Verification items for the finished model (mm, model axes). A direction names the side the tool comes from. Give positions to 0.01 mm unless a question says otherwise; leave off trailing zeros. Order: outer loops, then holes, each group sorted by start corner. A loop starts at its lowest first (then second) coordinate and runs counter-clockwise, first axis right, second up. Notation, with made-up numbers: (-6.5, 83.25) -> (-2.5, 83.25) arc R24 cw to (-2.5, 109.25) -> close; hole circle Ø9 at (-0.5, 12.5). An arc over 180 degrees is marked (long way). Write each question's results on one line, items separated by ' | '. Start each with the question number.
1. Cross-section at A-A, the plane y = 0. Enter the section's corners in (x, z) (3 decimals), then the cut area to 3 significant figures.
2. Material ranges on L1, parallel to Z at x = -12.5, y = -21.5; L2, parallel to X at y = -24.5, z = 62.5; L3, parallel to X at y = 35.5, z = 1, recorded low to high. Write a range as from..to.
3. Cross-section at B-B, the plane x = 30. Enter the section's corners in (y, z).
4. Depth check by flat-ended pin: pin 1 Ø16 at (y, z) = (0, 50.07) entering from +X; pin 2 Ø8 at (x, y) = (32, -9.5) entering from +Z; pin 3 Ø5 at (y, z) = (30, 75.07) entering from +X. Enter the tip coordinate at first touch or a pass-through.
5. Cross-section at C-C, the plane y = 30. Enter the section's corners in (x, z) (3 decimals), then the cut area to 3 significant figures.
6. Set-up check for faces 5 (the face through (-46.962, 9, 51)), 6 (the face through (2, 1, -3.038)): record each of +Z, -Z, +X, -X, +Y, -Y from which the full face is reachable in a straight line by a thin tool's end or side.
7. Mould release check, pull along X, two halves, no side actions. Record for faces 1 (the face through (-48.502, 22.968, 55.934)), 2 (the face through (-50, 9, 49)), 3 (the face through (26.746, -32.495, -1.498)), 4 (the face through (50, -1, -1)): +X half, -X half, draft (parallel to the pull), parting line (faces both ways), or undercut.
8. Cross-section at D-D, the plane y = 11.5. Enter the section's corners in (x, z) (3 decimals), then the cut area to 3 significant figures.
from build123d import *

# Parameters (mm, degrees)
CROQUIS1_W                       = 100
CROQUIS1_H                       = 80
CROQUIS1_R                       = 4.1
BRIDA_BASE1_DEPTH                = 3.03784
BRIDA_DE_ARISTA1_STRIP_W         = 18.50136
BRIDA_DE_ARISTA1_STRIP_H         = 3.03784
BRIDA_DE_ARISTA1_STRIP_CUT_DEPTH = 80
BRIDA_DE_ARISTA1_DEPTH           = 80
CORTAR_EXTRUIR1_REACH            = 146.919
CROQUIS9_R                       = 6.35
CROQUIS9_R_2                     = 3.1
CROQUIS9_R_3                     = 5


# Sheet-metal steps are written as plain solids
with BuildPart() as part:
    # Croquis1 → Brida base1 (new body)
    with BuildSketch(Plane.XY):
        Rectangle(CROQUIS1_W, CROQUIS1_H)
        with Locations((-30, 10)):
            Circle(CROQUIS1_R, mode=Mode.SUBTRACT)
        with Locations((30, 10)):
            Circle(CROQUIS1_R, mode=Mode.SUBTRACT)
        with Locations((-30, -30)):
            Circle(CROQUIS1_R, mode=Mode.SUBTRACT)
        with Locations((30, -30)):
            Circle(CROQUIS1_R, mode=Mode.SUBTRACT)
    extrude(amount=-BRIDA_BASE1_DEPTH)

    # Brida de arista1 strip (across the edge) → Brida de arista1 strip cut (cut)
    with BuildSketch(Plane(origin=(-50, 40, 0), x_dir=(1, 0, 0), z_dir=(0, -1, 0))):
        with Locations((-3.03784, -1.51892)):
            Rectangle(BRIDA_DE_ARISTA1_STRIP_W, BRIDA_DE_ARISTA1_STRIP_H)
    extrude(amount=BRIDA_DE_ARISTA1_STRIP_CUT_DEPTH, mode=Mode.SUBTRACT)

    # Brida de arista1 section (across the edge) → Brida de arista1 (add)
    with BuildSketch(Plane(origin=(-50, 40, 0), x_dir=(1, 0, 0), z_dir=(0, -1, 0))):
        with BuildLine():
            Line((0, 3.175), (0, 96.96216))
            Line((0, 96.96216), (3.03784, 96.96216))
            Line((3.03784, 96.96216), (3.03784, 3.175))
            ThreePointArc((3.03784, 3.175), (3.96777597, 0.92993597), (6.21284, 0))
            Line((6.21284, 0), (6.21284, -3.03784))
            ThreePointArc((6.21284, -3.03784), (1.819698706, -1.218141294), (0, 3.175))
        make_face()
    extrude(amount=BRIDA_DE_ARISTA1_DEPTH)

    # Croquis9 → Cortar-Extruir1 (cut, up to next)
    with BuildSketch(Plane.ZY.offset(50), mode=Mode.PRIVATE) as cortar_extruir1_sk1:
        with Locations((50.06858, 25.4)):
            Circle(CROQUIS9_R)
    cortar_extruir1_tool1 = extrude(cortar_extruir1_sk1.sketch, amount=-CORTAR_EXTRUIR1_REACH, mode=Mode.PRIVATE) & part.part
    # Croquis9 → Cortar-Extruir1 (cut, up to next)
    with BuildSketch(Plane.ZY.offset(50), mode=Mode.PRIVATE) as cortar_extruir1_sk2:
        with Locations((50.06858, -25.4)):
            Circle(CROQUIS9_R)
    cortar_extruir1_tool2 = extrude(cortar_extruir1_sk2.sketch, amount=-CORTAR_EXTRUIR1_REACH, mode=Mode.PRIVATE) & part.part
    # Croquis9 → Cortar-Extruir1 (cut, up to next)
    with BuildSketch(Plane.ZY.offset(50), mode=Mode.PRIVATE) as cortar_extruir1_sk3:
        with Locations((25.06858, 30)):
            Circle(CROQUIS9_R_2)
    cortar_extruir1_tool3 = extrude(cortar_extruir1_sk3.sketch, amount=-CORTAR_EXTRUIR1_REACH, mode=Mode.PRIVATE) & part.part
    # Croquis9 → Cortar-Extruir1 (cut, up to next)
    with BuildSketch(Plane.ZY.offset(50), mode=Mode.PRIVATE) as cortar_extruir1_sk4:
        with Locations((75.06858, 30)):
            Circle(CROQUIS9_R_2)
    cortar_extruir1_tool4 = extrude(cortar_extruir1_sk4.sketch, amount=-CORTAR_EXTRUIR1_REACH, mode=Mode.PRIVATE) & part.part
    # Croquis9 → Cortar-Extruir1 (cut, up to next)
    with BuildSketch(Plane.ZY.offset(50), mode=Mode.PRIVATE) as cortar_extruir1_sk5:
        with Locations((25.06858, -35)):
            Circle(CROQUIS9_R_2)
    cortar_extruir1_tool5 = extrude(cortar_extruir1_sk5.sketch, amount=-CORTAR_EXTRUIR1_REACH, mode=Mode.PRIVATE) & part.part
    # Croquis9 → Cortar-Extruir1 (cut, up to next)
    with BuildSketch(Plane.ZY.offset(50), mode=Mode.PRIVATE) as cortar_extruir1_sk6:
        with Locations((75.06858, -35)):
            Circle(CROQUIS9_R_2)
    cortar_extruir1_tool6 = extrude(cortar_extruir1_sk6.sketch, amount=-CORTAR_EXTRUIR1_REACH, mode=Mode.PRIVATE) & part.part
    # Croquis9 → Cortar-Extruir1 (cut, up to next)
    with BuildSketch(Plane.ZY.offset(50), mode=Mode.PRIVATE) as cortar_extruir1_sk7:
        with Locations((50.06858, 0)):
            Circle(CROQUIS9_R_3)
    cortar_extruir1_tool7 = extrude(cortar_extruir1_sk7.sketch, amount=-CORTAR_EXTRUIR1_REACH, mode=Mode.PRIVATE) & part.part
    add(cortar_extruir1_tool1.solids().sort_by_distance((-50, 25.4, 50.06858))[0], mode=Mode.SUBTRACT)
    add(cortar_extruir1_tool2.solids().sort_by_distance((-50, -25.4, 50.06858))[0], mode=Mode.SUBTRACT)
    add(cortar_extruir1_tool3.solids().sort_by_distance((-50, 30, 25.06858))[0], mode=Mode.SUBTRACT)
    add(cortar_extruir1_tool4.solids().sort_by_distance((-50, 30, 75.06858))[0], mode=Mode.SUBTRACT)
    add(cortar_extruir1_tool5.solids().sort_by_distance((-50, -35, 25.06858))[0], mode=Mode.SUBTRACT)
    add(cortar_extruir1_tool6.solids().sort_by_distance((-50, -35, 75.06858))[0], mode=Mode.SUBTRACT)
    add(cortar_extruir1_tool7.solids().sort_by_distance((-50, 0, 50.06858))[0], mode=Mode.SUBTRACT)


solid = part.part
Results below:
1) outline: (-50, 3.175) arc R6.213 ccw to (-43.787, -3.038) -> (50, -3.038) -> (50, 0) -> (-43.787, 0) arc R3.175 cw to (-46.962, 3.175) -> (-46.962, 45.069) -> (-50, 45.069) -> close; (-50, 55.069) -> (-46.962, 55.069) -> (-46.962, 96.962) -> (-50, 96.962) -> close | area: 562 mm²
2) L1: z = -3.04..0 | L2: x = -50..-46.96 | L3: x = -49.61..-46.1
3) outline: (-40, -3.04) -> (-34.1, -3.04) -> (-34.1, 0) -> (-40, 0) -> close; (-25.9, -3.04) -> (5.9, -3.04) -> (5.9, 0) -> (-25.9, 0) -> close; (14.1, -3.04) -> (40, -3.04) -> (40, 0) -> (14.1, 0) -> close
4) pin 1: stops at x = -46.96 | pin 2: stops at z = 0 | pin 3: passes through
5) outline: (-50, 3.175) arc R6.213 ccw to (-43.787, -3.038) -> (50, -3.038) -> (50, 0) -> (-43.787, 0) arc R3.175 cw to (-46.962, 3.175) -> (-46.962, 21.969) -> (-50, 21.969) -> close; (-50, 28.169) -> (-46.962, 28.169) -> (-46.962, 45.691) -> (-50, 45.691) -> close; (-50, 54.446) -> (-46.962, 54.446) -> (-46.962, 71.969) -> (-50, 71.969) -> close; (-50, 78.169) -> (-46.962, 78.169) -> (-46.962, 96.962) -> (-50, 96.962) -> close | area: 528 mm²
6) face 5: +Z, +X, +Y, -Y | face 6: -Z, +X, -X, +Y, -Y
7) face 1: draft | face 2: -X half | face 3: undercut | face 4: +X half
8) outline: (-50, 3.175) arc R6.213 ccw to (-43.787, -3.038) -> (-33.816, -3.038) -> (-33.816, 0) -> (-43.787, 0) arc R3.175 cw to (-46.962, 3.175) -> (-46.962, 96.962) -> (-50, 96.962) -> close; (-26.184, -3.038) -> (26.184, -3.038) -> (26.184, 0) -> (-26.184, 0) -> close; (33.816, -3.038) -> (50, -3.038) -> (50, 0) -> (33.816, 0) -> close | area: 546 mm²
